Verification items for the finished model (mm, model axes). A direction names the side the tool comes from. Round coordinates to 2 decimals unless told otherwise and drop trailing zeros. Loops run counter-clockwise (first coordinate to the right, second up) from the corner with the lowest first, then second, coordinate; pieces in that order, holes last. Notation, with made-up numbers: (27, -26.75) - (37, -26.75) arc R5 cw to (37, -18.75) - close; hole circle Ø9 at (-30.75, 81.5). An arc over 180 degrees is marked (long way). Use a Markdown table: item, result. Add a question column.
```python
from build123d import *

# Parameters (mm, degrees)
BODY_DEPTH                 = 15
SKETCH3_W                  = 2
SKETCH3_H                  = 15
SKETCH3_W_2                = 15
SKETCH3_H_2                = 2
FIELD_CUT_DEPTH            = 2
FIELD_CHAMFER_SIZE         = 2
CLICK_CHAMFER_1_DEPTH      = 225.199687779
CLICK_CHAMFER_1_DEPTH_BACK = 225.199687779
CLICK_CHAMFER_2_DEPTH      = 225.199687779
CLICK_CHAMFER_2_DEPTH_BACK = 225.199687779
SKETCH7_R                  = 2.5
LED_HOLE_2_DEPTH           = 8
SKETCH8_R                  = 2.5
LED_HOLE_1_DEPTH           = 8
CORNER_CHAMFER_DEPTH       = 214.367054627
CORNER_CHAMFER_DEPTH_BACK  = 214.367054627
CLICK_HOLE_DEPTH           = 7.5
SKETCH12_W                 = 1
SKETCH12_H                 = 15
LIGHT_GUIDE_1_DEPTH        = 13
SKETCH13_W                 = 15
SKETCH13_H                 = 1
LIGHT_GUIDE_2_DEPTH        = 13
MOUNTING_HOLE_DEPTH        = 214.367054627
MOUNTING_HOLE_DEPTH_BACK   = 214.367054627
SKETCH14_R                 = 1.75
SKETCH15_W                 = 1
SKETCH15_H                 = 19
SKETCH15_W_2               = 19
SKETCH15_H_2               = 1
CUT_EXTRUDE1_DEPTH         = 13.25


with BuildPart() as part:
    # Sketch1 → Body (new body)
    with BuildSketch(Plane.XY):
        Polygon((0, 0), (0, 150.5), (15, 150.5), (15, -15), (-150.5, -15), (-150.5, 0), align=None)
    extrude(amount=BODY_DEPTH)

    # Sketch3 → Field Cut (cut)
    with BuildSketch(Plane.XY.offset(15)):
        with Locations((-50.25, -7.5)):
            Rectangle(SKETCH3_W, SKETCH3_H)
        with Locations((-100.5, -7.5)):
            Rectangle(SKETCH3_W, SKETCH3_H)
        with Locations((7.5, 50.25)):
            Rectangle(SKETCH3_W_2, SKETCH3_H_2)
        with Locations((7.5, 100.5)):
            Rectangle(SKETCH3_W_2, SKETCH3_H_2)
    extrude(amount=-FIELD_CUT_DEPTH, mode=Mode.SUBTRACT)

    # Field Chamfer
    # the kernel refuses this chamfer: 2 mm, written as the material it adds along each edge
    with BuildSketch(Plane(origin=(-101.5, 0, 13), x_dir=(0.9996219169112968, 0, -0.027495876610586414), z_dir=(0, -1, 0))) as field_chamfer_piece_1_section:
        Polygon((FIELD_CHAMFER_SIZE * 0.999621916911, FIELD_CHAMFER_SIZE * 0.0274958766106), (-FIELD_CHAMFER_SIZE * 0.0274958766106, FIELD_CHAMFER_SIZE * 0.999621916911), (0, 0), align=None)
    field_chamfer_piece_1 = extrude(amount=15, mode=Mode.PRIVATE)
    field_chamfer_piece_1 = split(field_chamfer_piece_1, bisect_by=Plane(origin=(-100.839191691, -7.5, 15), z_dir=(0, 0, -1)), keep=Keep.TOP, mode=Mode.PRIVATE)
    add(field_chamfer_piece_1)
    with BuildSketch(Plane(origin=(-99.5, -15, 13), x_dir=(0.02749587661058907, 0, 0.9996219169112965), z_dir=(0, 1, 0))) as field_chamfer_piece_2_section:
        Polygon((FIELD_CHAMFER_SIZE * 0.999621916911, -FIELD_CHAMFER_SIZE * 0.0274958766106), (-FIELD_CHAMFER_SIZE * 0.0274958766106, -FIELD_CHAMFER_SIZE * 0.999621916911), (0, 0), align=None)
    field_chamfer_piece_2 = extrude(amount=15, mode=Mode.PRIVATE)
    field_chamfer_piece_2 = split(field_chamfer_piece_2, bisect_by=Plane(origin=(-100.160808309, -7.5, 15), z_dir=(0, 0, -1)), keep=Keep.TOP, mode=Mode.PRIVATE)
    add(field_chamfer_piece_2)
    with BuildSketch(Plane(origin=(-51.25, 0, 13), x_dir=(0.9996219169112968, 0, -0.02749587661058651), z_dir=(0, -1, 0))) as field_chamfer_piece_3_section:
        Polygon((FIELD_CHAMFER_SIZE * 0.999621916911, FIELD_CHAMFER_SIZE * 0.0274958766106), (-FIELD_CHAMFER_SIZE * 0.0274958766106, FIELD_CHAMFER_SIZE * 0.999621916911), (0, 0), align=None)
    field_chamfer_piece_3 = extrude(amount=15, mode=Mode.PRIVATE)
    field_chamfer_piece_3 = split(field_chamfer_piece_3, bisect_by=Plane(origin=(-50.589191691, -7.5, 15), z_dir=(0, 0, -1)), keep=Keep.TOP, mode=Mode.PRIVATE)
    add(field_chamfer_piece_3)
    with BuildSketch(Plane(origin=(-49.25, -15, 13), x_dir=(0.027495876610585623, 0, 0.9996219169112968), z_dir=(0, 1, 0))) as field_chamfer_piece_4_section:
        Polygon((FIELD_CHAMFER_SIZE * 0.999621916911, -FIELD_CHAMFER_SIZE * 0.0274958766106), (-FIELD_CHAMFER_SIZE * 0.0274958766106, -FIELD_CHAMFER_SIZE * 0.999621916911), (0, 0), align=None)
    field_chamfer_piece_4 = extrude(amount=15, mode=Mode.PRIVATE)
    field_chamfer_piece_4 = split(field_chamfer_piece_4, bisect_by=Plane(origin=(-49.910808309, -7.5, 15), z_dir=(0, 0, -1)), keep=Keep.TOP, mode=Mode.PRIVATE)
    add(field_chamfer_piece_4)
    with BuildSketch(Plane(origin=(15, 49.25, 13), x_dir=(0, 0.9996219169112968, -0.02749587661058651), z_dir=(-1, 0, 0))) as field_chamfer_piece_5_section:
        Polygon((FIELD_CHAMFER_SIZE * 0.999621916911, -FIELD_CHAMFER_SIZE * 0.0274958766106), (-FIELD_CHAMFER_SIZE * 0.0274958766106, -FIELD_CHAMFER_SIZE * 0.999621916911), (0, 0), align=None)
    field_chamfer_piece_5 = extrude(amount=15, mode=Mode.PRIVATE)
    field_chamfer_piece_5 = split(field_chamfer_piece_5, bisect_by=Plane(origin=(7.5, 49.910808309, 15), z_dir=(0, 0, -1)), keep=Keep.TOP, mode=Mode.PRIVATE)
    add(field_chamfer_piece_5)
    with BuildSketch(Plane(origin=(0, 51.25, 13), x_dir=(0, 0.027495876610585623, 0.9996219169112968), z_dir=(1, 0, 0))) as field_chamfer_piece_6_section:
        Polygon((FIELD_CHAMFER_SIZE * 0.999621916911, FIELD_CHAMFER_SIZE * 0.0274958766106), (-FIELD_CHAMFER_SIZE * 0.0274958766106, FIELD_CHAMFER_SIZE * 0.999621916911), (0, 0), align=None)
    field_chamfer_piece_6 = extrude(amount=15, mode=Mode.PRIVATE)
    field_chamfer_piece_6 = split(field_chamfer_piece_6, bisect_by=Plane(origin=(7.5, 50.589191691, 15), z_dir=(0, 0, -1)), keep=Keep.TOP, mode=Mode.PRIVATE)
    add(field_chamfer_piece_6)
    with BuildSketch(Plane(origin=(0, 101.5, 13), x_dir=(0, 0.02749587661058907, 0.9996219169112965), z_dir=(1, 0, 0))) as field_chamfer_piece_7_section:
        Polygon((FIELD_CHAMFER_SIZE * 0.999621916911, FIELD_CHAMFER_SIZE * 0.0274958766106), (-FIELD_CHAMFER_SIZE * 0.0274958766106, FIELD_CHAMFER_SIZE * 0.999621916911), (0, 0), align=None)
    field_chamfer_piece_7 = extrude(amount=15, mode=Mode.PRIVATE)
    field_chamfer_piece_7 = split(field_chamfer_piece_7, bisect_by=Plane(origin=(7.5, 100.839191691, 15), z_dir=(0, 0, -1)), keep=Keep.TOP, mode=Mode.PRIVATE)
    add(field_chamfer_piece_7)
    with BuildSketch(Plane(origin=(15, 99.5, 13), x_dir=(0, 0.9996219169112968, -0.027495876610586414), z_dir=(-1, 0, 0))) as field_chamfer_piece_8_section:
        Polygon((FIELD_CHAMFER_SIZE * 0.999621916911, -FIELD_CHAMFER_SIZE * 0.0274958766106), (-FIELD_CHAMFER_SIZE * 0.0274958766106, -FIELD_CHAMFER_SIZE * 0.999621916911), (0, 0), align=None)
    field_chamfer_piece_8 = extrude(amount=15, mode=Mode.PRIVATE)
    field_chamfer_piece_8 = split(field_chamfer_piece_8, bisect_by=Plane(origin=(7.5, 100.160808309, 15), z_dir=(0, 0, -1)), keep=Keep.TOP, mode=Mode.PRIVATE)
    add(field_chamfer_piece_8)

    # Sketch4 → Click Chamfer 1 (cut, two sides: drawn at the far end of the back side and taken through both)
    with BuildSketch(Plane.XZ.offset(15).offset(-CLICK_CHAMFER_1_DEPTH_BACK)):
        Polygon((-150.5, 15), (-150.5, 14), (-149.5, 15), align=None)
    extrude(amount=CLICK_CHAMFER_1_DEPTH + CLICK_CHAMFER_1_DEPTH_BACK, mode=Mode.SUBTRACT)

    # Sketch5 → Click Chamfer 2 (cut, two sides: drawn at the far end of the back side and taken through both)
    with BuildSketch(Plane(origin=(15, 0, 0), x_dir=(0, 0, -1), z_dir=(1, 0, 0)).offset(-CLICK_CHAMFER_2_DEPTH_BACK)):
        Polygon((-15, 150.5), (-15, 149.5), (-14, 150.5), align=None)
    extrude(amount=CLICK_CHAMFER_2_DEPTH + CLICK_CHAMFER_2_DEPTH_BACK, mode=Mode.SUBTRACT)

    # Sketch7 → LED Hole 2 (cut)
    with BuildSketch(Plane.ZY):
        with Locations((5.75, 75.25)):
            Circle(SKETCH7_R)
        with Locations((5.75, 125.5)):
            Circle(SKETCH7_R)
        with Locations((5.75, 25.25)):
            Circle(SKETCH7_R)
    extrude(amount=-LED_HOLE_2_DEPTH, mode=Mode.SUBTRACT)

    # Sketch8 → LED Hole 1 (cut)
    with BuildSketch(Plane(origin=(0, 0, 0), x_dir=(1, 0, 0), z_dir=(0, 1, 0))):
        with Locations(Location((-125.5, -5.75, 0), (0, 0, 270))):
            Circle(SKETCH8_R)
        with Locations(Location((-75.5, -5.75, 0), (0, 0, 270))):
            Circle(SKETCH8_R)
        with Locations(Location((-25.25, -5.75, 0), (0, 0, 270))):
            Circle(SKETCH8_R)
    extrude(amount=-LED_HOLE_1_DEPTH, mode=Mode.SUBTRACT)

    # Sketch9 → Corner Chamfer (cut, two sides: drawn at the far end of the back side and taken through both)
    with BuildSketch(Plane.XY.offset(15).offset(-CORNER_CHAMFER_DEPTH_BACK)):
        Polygon((15, -6.213203436), (6.213203436, -15), (15, -15), align=None)
    extrude(amount=CORNER_CHAMFER_DEPTH + CORNER_CHAMFER_DEPTH_BACK, mode=Mode.SUBTRACT)

    # Sketch10 → Click Hole (cut)
    with BuildSketch(Plane(origin=(0, 0, 0), x_dir=(-1, 0, 0), z_dir=(0, 0, -1))):
        Polygon((150.5, -5), (143, -2.5), (143, -12.5), (150.5, -10), align=None)
        Polygon((-7.5, 150.5), (-10, 150.5), (-12.5, 143), (-7.5, 143), (-2.5, 143), (-5, 150.5), align=None)
    extrude(amount=-CLICK_HOLE_DEPTH, mode=Mode.SUBTRACT)

    # Sketch12 → Light Guide 1 (cut)
    with BuildSketch(Plane(origin=(0, -1, 0), x_dir=(1, 0, 0), z_dir=(0, 1, 0))):
        with Locations((-35.25, -5.75)):
            Rectangle(SKETCH12_W, SKETCH12_H)
        with Locations((-15.25, -5.75)):
            Rectangle(SKETCH12_W, SKETCH12_H)
        with Locations((-65.5, -5.75)):
            Rectangle(SKETCH12_W, SKETCH12_H)
        with Locations((-85.5, -5.75)):
            Rectangle(SKETCH12_W, SKETCH12_H)
        with Locations((-115.5, -5.75)):
            Rectangle(SKETCH12_W, SKETCH12_H)
        with Locations((-135.5, -5.75)):
            Rectangle(SKETCH12_W, SKETCH12_H)
    extrude(amount=-LIGHT_GUIDE_1_DEPTH, mode=Mode.SUBTRACT)

    # Sketch13 → Light Guide 2 (cut)
    with BuildSketch(Plane.ZY.offset(-1)):
        with Locations((5.75, 35.25)):
            Rectangle(SKETCH13_W, SKETCH13_H)
        with Locations((5.75, 15.25)):
            Rectangle(SKETCH13_W, SKETCH13_H)
        with Locations((5.75, 65.25)):
            Rectangle(SKETCH13_W, SKETCH13_H)
        with Locations((5.75, 85.25)):
            Rectangle(SKETCH13_W, SKETCH13_H)
        with Locations((5.75, 115.5)):
            Rectangle(SKETCH13_W, SKETCH13_H)
        with Locations((5.75, 135.5)):
            Rectangle(SKETCH13_W, SKETCH13_H)
    extrude(amount=-LIGHT_GUIDE_2_DEPTH, mode=Mode.SUBTRACT)

    # Sketch14 → Mounting Hole (cut, two sides: drawn at the far end of the back side and taken through both)
    with BuildSketch(Plane.XY.offset(15).offset(-MOUNTING_HOLE_DEPTH_BACK)):
        with Locations((5.303300859, -5.303300859)):
            Circle(SKETCH14_R)
    extrude(amount=MOUNTING_HOLE_DEPTH + MOUNTING_HOLE_DEPTH_BACK, mode=Mode.SUBTRACT)

    # Sketch15 → Cut-Extrude1 (cut)
    with BuildSketch(Plane(origin=(0, 0, 0), x_dir=(-1, 0, 0), z_dir=(0, 0, -1))):
        with Locations((-13.5, 125.5)):
            Rectangle(SKETCH15_W, SKETCH15_H)
        with Locations((-13.5, 75.25)):
            Rectangle(SKETCH15_W, SKETCH15_H)
        with Locations((-13.5, 25.25)):
            Rectangle(SKETCH15_W, SKETCH15_H)
        with Locations((25.25, -13.5)):
            Rectangle(SKETCH15_W_2, SKETCH15_H_2)
        with Locations((75.5, -13.5)):
            Rectangle(SKETCH15_W_2, SKETCH15_H_2)
        with Locations((125.5, -13.5)):
            Rectangle(SKETCH15_W_2, SKETCH15_H_2)
    extrude(amount=-CUT_EXTRUDE1_DEPTH, mode=Mode.SUBTRACT)


solid = part.part
```
Q1. Thickness scan on line 1 along Y through (x, z) = (-33.5, 5.25); line 2 along X through (y, z) = (82, 12.5); line 3 along Z through (x, y) = (4, 25). Record the ranges inside material, lowest first.
Q2. Section check D-D on z = 5.5. State how many separate pieces and enclosed holes the cut face has, plus the area to 3 significant figures.
Q3. Section check B-B on y = 82. Record the cut outline in (x, z).
Q4. Section check C-C on y = 125.5. Record the cut outline in (x, z).
Q5. Release check for a two-part mould opening along X. For faces 5 (the face through (7, 116, 7)), 6 (the face through (8, 75, 6)), 7 (the face through (-125, -7, 15)) record: +X half, -X half, draft (parallel to the pull), parting line (faces both ways), or undercut.
Q6. Set-up check for faces 1 (the face through (-25, -8, 6)), 2 (the face through (3.94, 73.03, 6.9)), 3 (the face through (-150.5, -8, 8)), 4 (the face through (-66, -7, 7)): record each of +Z, -Z, +X, -X, +Y, -Y from which the full face is reachable in a straight line by a thin tool's end or side.
Q7. Go/stop test with flat-tipped pins: pin 1 Ø6.5 at (y, z) = (70.5, 7) entering from -X; pin 2 Ø2 at (x, z) = (8, 2.5) entering from +Y; pin 3 Ø1.5 at (x, z) = (-124.5, 6.5) entering from +Y. Record where each tip stops, or that it passes through.
Q8. Section check A-A on x = -75.5. Record the cut outline in (y, z).
Determined:
| question | item | result |
|---|---|---|
| 1 | line 1 | y = -15 to -14, -13 to 0 |
| 1 | line 2 | x = 0 to 13, 14 to 15 |
| 1 | line 3 | z = 0 to 3.26, 8.24 to 15 |
| 2 | separate pieces | 1 |
| 2 | enclosed holes | 7 |
| 2 | area | 4,070 mm² |
| 3 | outline | (0, 0) - (13, 0) - (13, 13.25) - (14, 13.25) - (14, 0) - (15, 0) - (15, 15) - (0, 15) - close |
| 4 | outline | (0, 0) - (13, 0) - (13, 13.25) - (14, 13.25) - (14, 0) - (15, 0) - (15, 15) - (0, 15) - (0, 8.25) - (8, 8.25) - (8, 3.25) - (0, 3.25) - close |
| 5 | face 5 | undercut |
| 5 | face 6 | -X half |
| 5 | face 7 | draft |
| 6 | face 1 | +Y |
| 6 | face 2 | -X |
| 6 | face 3 | +Z, -Z, -X, +Y, -Y |
| 6 | face 4 | -Z |
| 7 | pin 1 | stops at x = 0 |
| 7 | pin 2 | stops at y = 143 |
| 7 | pin 3 | stops at y = -8 |
| 8 | outline | (-15, 0) - (-14, 0) - (-14, 13.25) - (-13, 13.25) - (-13, 0) - (0, 0) - (0, 3.25) - (-8, 3.25) - (-8, 8.25) - (0, 8.25) - (0, 15) - (-15, 15) - close |
